Can you work these out from the model? Positions are in its coordinate system, mm. Face numbers are marked on the shaded views. A direction names the side the tool comes from. Round coordinates to 2 decimals unless told otherwise and drop trailing zeros. Loops run counter-clockwise (first coordinate to the right, second up) from the corner with the lowest first, then second, coordinate; pieces in that order, holes last.
from build123d import *

# Parameters (mm, degrees)
BOSS_EXTRUDE1_DEPTH = 20
SKETCH2_W           = 0.8000000000000007
SKETCH2_H           = 0.7999999999999989
SKETCH2_H_2         = 0.8000000000000007
CHAMFER1_SIZE       = 0.4
FILLET2_R           = 2
SKETCH3_R           = 2.100000000000004
SKETCH3_R_2         = 2.100000000000001
CUT_EXTRUDE1_DEPTH  = 44.163354633534205
SKETCH4_R           = 3.7499999999999996
SKETCH4_R_2         = 3.750000000000006
CUT_EXTRUDE2_DEPTH  = 5


# Some blends are built 0.0001 mm under size
with BuildPart() as part:
    # Sketch1 → Boss-Extrude1 (new body)
    with BuildSketch(Plane.XY):
        with BuildLine():
            Line((0.9198479389646088, 12.89190109356241), (0.9198479389646088, 2.89190109356241))
            Line((0.9198479389646081, 2.89190109356241), (8.919847938964608, 2.89190109356241))
            ThreePointArc((8.919847938964608, 2.8919010935624105), (10.919847938964608, 4.89190109356241), (12.919847938964608, 2.89190109356241))
            Line((12.919847938964608, 2.89190109356241), (13.669847938964606, 2.89190109356241))
            ThreePointArc((13.669847938964608, 2.8919010935624114), (18.919847938964608, 8.14190109356241), (24.169847938964608, 2.89190109356241))
            Line((24.169847938964608, 2.89190109356241), (24.919847938964608, 2.89190109356241))
            ThreePointArc((24.919847938964608, 2.8919010935624105), (26.919847938964608, 4.891901093562406), (28.919847938964608, 2.89190109356241))
            Line((28.919847938964605, 2.89190109356241), (36.91984793896461, 2.89190109356241))
            Line((36.91984793896461, 2.89190109356241), (36.91984793896461, 12.89190109356241))
            Line((36.91984793896461, 12.89190109356241), (0.9198479389646088, 12.89190109356241))
        make_face()
    extrude(amount=BOSS_EXTRUDE1_DEPTH)

    # Sweep2: sweep along a curve in space
    with BuildLine() as sweep2_path:
        ThreePointArc((24.169847938964608, 2.89190109356241, 20), (22.632158540193984, 6.604211694791784, 20), (18.919847938964608, 8.141901093562412, 20))
        ThreePointArc((18.919847938964608, 8.141901093562412, 20), (15.207537337735232, 6.604211694791786, 20), (13.669847938964606, 2.89190109356241, 20))
    # Sketch2 → Sweep2 (sweep)
    with BuildSketch(Plane.XZ.offset(-2.89190109356241)):
        with Locations((14.069847938964607, 13.400000000000006)):
            Rectangle(SKETCH2_W, SKETCH2_H)
        with Locations((14.069847938964607, 10.400000000000004)):
            Rectangle(SKETCH2_W, SKETCH2_H_2)
        with Locations((14.069847938964607, 7.400000000000003)):
            Rectangle(SKETCH2_W, SKETCH2_H_2)
        Polygon((13.669847938964608, 4.8000000000000025), (14.469847938964607, 4.8000000000000025), (14.469847938964609, 4.000000000000002), (13.669847938964608, 4.000000000000002), align=None)
    sweep(path=sweep2_path.line)

    # Chamfer1
    chamfer1_edges = [part.edges().sort_by_distance(p)[0] for p in [
        (18.919847938964608, 7.341901093562408, 4.000000000000002),
        (18.919847938964608, 7.341901093562411, 4.8000000000000025),
        (18.919847938964608, 7.341901093562411, 7.0000000000000036),
        (18.919847938964608, 7.341901093562413, 7.800000000000004),
        (18.919847938964608, 7.341901093562413, 13.800000000000004),
        (18.919847938964608, 7.341901093562411, 13.000000000000005),
        (18.919847938964608, 7.341901093562413, 10.800000000000004),
        (18.919847938964608, 7.341901093562411, 10.000000000000004),
    ]]
    chamfer(chamfer1_edges, length=CHAMFER1_SIZE - 0.0001)  # a hair under: the kernel refuses the full size

    # Fillet2
    # the kernel refuses this fillet: 2 mm, written as the material it takes off along each edge
    with BuildSketch(Plane(origin=(10.919847938964608, 2.89190109356241, 0), x_dir=(-0.003141587485879782, -0.9999950652018582, 0), z_dir=(0.9999950652018582, -0.003141587485879782, 0))) as fillet2_piece_1:
        with BuildLine():
            CenterArc((2 + FILLET2_R, -FILLET2_R), FILLET2_R, 89.99999999999997, 90)
            Line((2 + FILLET2_R, 2.2e-16), (2, 0))
            Line((2, 0), (2, -FILLET2_R))
        make_face()
    revolve(axis=Axis((10.919847938964608, 2.89190109356241, 0), (0, 0, -1)), revolution_arc=359.64000000000004, mode=Mode.SUBTRACT)
    with BuildSketch(Plane(origin=(26.919847938964608, 2.8919010935624057, 0), x_dir=(-0.003141587485879782, -0.9999950652018582, 0), z_dir=(0.9999950652018582, -0.003141587485879782, 0))) as fillet2_piece_2:
        with BuildLine():
            CenterArc((1.9999999999999987 + FILLET2_R, -FILLET2_R), FILLET2_R, 90, 90)
            Line((1.999999999999998, -FILLET2_R), (1.9999999999999987, 0))
            Line((1.9999999999999987, 0), (1.9999999999999987 + FILLET2_R, 0))
        make_face()
    revolve(axis=Axis((26.919847938964608, 2.8919010935624057, 0), (0, 0, -1)), revolution_arc=359.64, mode=Mode.SUBTRACT)
    with BuildSketch(Plane(origin=(10.919847938964608, 2.89190109356241, 20), x_dir=(-0.003141587485879782, -0.9999950652018582, 0), z_dir=(0.9999950652018582, -0.003141587485879782, 0))) as fillet2_piece_3:
        with BuildLine():
            CenterArc((1.9999999999999987 + FILLET2_R, FILLET2_R), FILLET2_R, 180, 90)
            Line((1.999999999999999, FILLET2_R), (1.9999999999999987, 0))
            Line((1.9999999999999987, 0), (1.9999999999999987 + FILLET2_R, 0))
        make_face()
    revolve(axis=Axis((10.919847938964608, 2.89190109356241, 20), (0, 0, -1)), revolution_arc=359.64000000000004, mode=Mode.SUBTRACT)
    with BuildSketch(Plane(origin=(26.919847938964608, 2.8919010935624057, 20), x_dir=(-0.003141587485879782, -0.9999950652018582, 0), z_dir=(0.9999950652018582, -0.003141587485879782, 0))) as fillet2_piece_4:
        with BuildLine():
            CenterArc((1.9999999999999987 + FILLET2_R, FILLET2_R), FILLET2_R, 180, 90)
            Line((1.999999999999998, FILLET2_R), (1.9999999999999987, 0))
            Line((1.9999999999999987, 0), (1.9999999999999987 + FILLET2_R, 0))
        make_face()
    revolve(axis=Axis((26.919847938964608, 2.8919010935624057, 20), (0, 0, -1)), revolution_arc=359.64, mode=Mode.SUBTRACT)

    # Sketch3 → Cut-Extrude1 (cut, through all)
    with BuildSketch(Plane.XZ.offset(-2.89190109356241)):
        with Locations(Location((32.9198479389646, 10, 0), (0, 0, 270))):
            Circle(SKETCH3_R)
        with Locations(Location((4.919847938964609, 10, 0), (0, 0, 270))):
            Circle(SKETCH3_R_2)
    extrude(amount=-CUT_EXTRUDE1_DEPTH, mode=Mode.SUBTRACT)

    # Sketch4 → Cut-Extrude2 (cut)
    with BuildSketch(Plane(origin=(0, 12.89190109356241, 0), x_dir=(1, 0, 0), z_dir=(0, 1, 0))):
        with Locations(Location((4.919847938964609, -10, 0), (0, 0, 270))):
            Circle(SKETCH4_R)
        with Locations(Location((32.9198479389646, -10, 0), (0, 0, 270))):
            Circle(SKETCH4_R_2)
    extrude(amount=-CUT_EXTRUDE2_DEPTH, mode=Mode.SUBTRACT)


solid = part.part
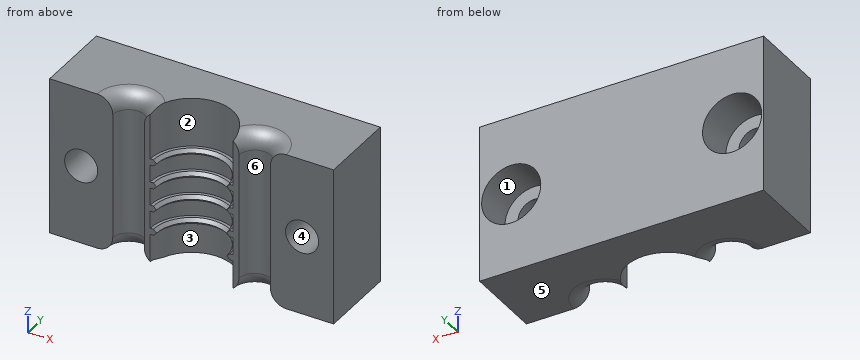
(1) If we section it at A-A, the plane z = 11.5: List the corners of the cut face in (x, y) for me.
Worked answers:
outline: (0.92, 2.89) - (3.45, 2.89) - (3.45, 7.89) - (1.48, 7.89) - (1.48, 12.89) - (0.92, 12.89) - close; (6.39, 2.89) - (8.92, 2.89) arc R2 cw to (12.92, 2.89) - (13.67, 2.89) arc R5.25 cw to (24.17, 2.89) - (24.92, 2.89) arc R2 cw to (28.92, 2.89) - (31.45, 2.89) - (31.45, 7.89) - (29.48, 7.89) - (29.48, 12.89) - (8.36, 12.89) - (8.36, 7.89) - (6.39, 7.89) - close; (34.39, 2.89) - (36.92, 2.89) - (36.92, 12.89) - (36.36, 12.89) - (36.36, 7.89) - (34.39, 7.89) - close
(2) If we mould it in two halves opening along Z, with no side actions, what happens to the marked faces 4, 5 and 6? For each: released by +Z, released by -Z, zero draft, split by the parting line, or undercut.
Worked answers:
face 4: undercut
face 5: released by -Z
face 6: zero draft
(3) For the marked faces 1, 2 and 3, which set-ups out of +Z, -Z, +X, -X, +Y, -Y let a thin tool reach every point of the face, with its end or its side?
Worked answers:
face 1: +Y
face 2: +Z, -Y
face 3: -Z, -Y
(4) Will these pins go through, and if not, where does the flat tip stop? P1, Ø6, axis at x = 20, y = 4.5, coming from the -Z side; P2, Ø2, axis at x = 5.5, z = 11, coming from the +Y side.
Worked answers:
P1: stops at z = 4
P2: stops at y = 7.89
(5) If I drill on line 1 (X direction, y = 9.5, z = 10); line 2 (X direction, y = 7.25, z = 11); line 3 (X direction, y = 9, z = 10.75), over which ranges is the centre line in solid material (lowest first)?
Worked answers:
line 1: x = 0.92 to 1.17, 8.67 to 29.17, 36.67 to 36.92
line 2: x = 0.92 to 3.07, 6.77 to 15.99, 21.85 to 31.07, 34.77 to 36.92
line 3: x = 0.92 to 1.25, 8.59 to 29.25, 36.59 to 36.92
(6) If we section it at C-C, the plane z = 17: List the corners of the cut face in (x, y) for me, then the cut area to 3 significant figures.
Worked answers:
outline: (0.92, 2.89) - (8.92, 2.89) arc R2 cw to (12.92, 2.89) - (13.67, 2.89) arc R5.25 cw to (24.17, 2.89) - (24.92, 2.89) arc R2 cw to (28.92, 2.89) - (36.92, 2.89) - (36.92, 12.89) - (0.92, 12.89) - close
area: 304 mm2
(7) If we section it at B-B, the plane y = 9.25: List the corners of the cut face in (x, z) for me.
Worked answers:
outline: (0.92, 0) - (36.92, 0) - (36.92, 20) - (0.92, 20) - close; hole circle Ø7.5 at (4.92, 10); hole circle Ø7.5 at (32.92, 10)
